Geometry check sheet. Reference: drawing and pictorial views, mm from the part's lowest x, y, z. Round coordinates to 2 decimals unless told otherwise and drop trailing zeros. Write each loop counter-clockwise with the first axis right and the second up, starting at its lowest first coordinate (ties: lowest second). Pieces come first, ordered by that corner, then holes. Notation, with made-up numbers: (22.5, -31.5) -> (31.5, -31.5) arc R12 cw to (31.5, -10.5) -> close; hole circle Ø9 at (69, -1). An arc over 180 degrees is marked (long way). Answer as a JSON object with one key per item and string values. Group by question number.
(1) Gauge pin test, flat ends, axial feed: pin 1 Ø1.2 at (x, z) = (45.5, 2.5) entering from -Y; pin 2 Ø1.2 at (y, z) = (1.5, 1) entering from +X; pin 3 Ø2 at (y, z) = (2.5, 3) entering from -X. Record the tip position at first contact, or that the pin passes through.
(2) Scan lines: L1, parallel to X at y = 17, z = 2.35; L2, parallel to Y at x = 53, z = 1.6; L3, parallel to Y at x = 24, z = 2. Record each from-to range of solid material in increasing order. Write a range as from..to.
(3) Sectioned sample at B-B on y = 16.5. Record the cut outline in (x, z), and give its area (3 significant figures).
(4) Sectioned sample at A-A on x = 18. Record the cut outline in (y, z), and give its area (3 significant figures).
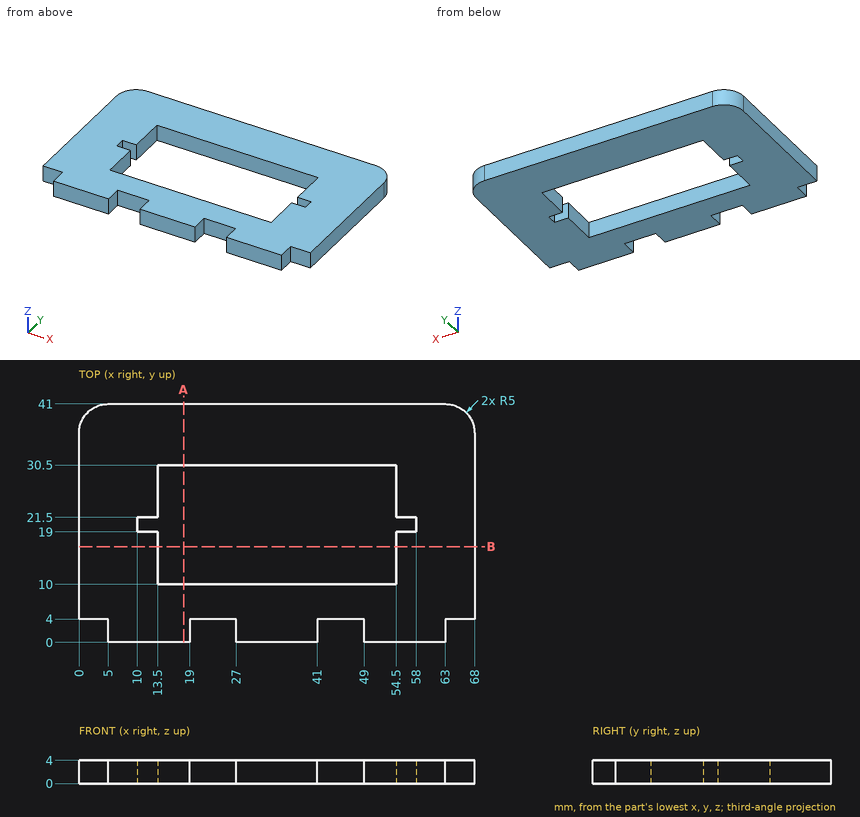
Computed values:
{
 "1": {"pin 1": "y = 4", "pin 2": "x = 63", "pin 3": "x = 5"},
 "2": {"L1": "0..13.5, 54.5..68", "L2": "0..10, 30.5..41", "L3": "4..10, 30.5..41"},
 "3": {"outline": "(0, 0) -> (13.5, 0) -> (13.5, 4) -> (0, 4) -> close; (54.5, 0) -> (68, 0) -> (68, 4) -> (54.5, 4) -> close", "area": "108 mm2"},
 "4": {"outline": "(0, 0) -> (10, 0) -> (10, 4) -> (0, 4) -> close; (30.5, 0) -> (41, 0) -> (41, 4) -> (30.5, 4) -> close", "area": "82.0 mm2"}
}
